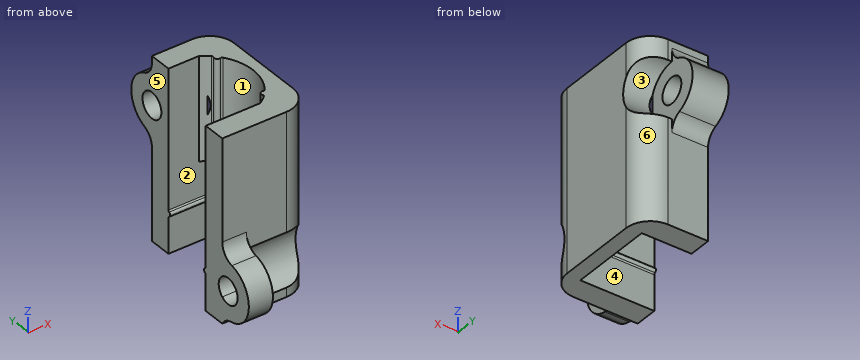
from build123d import *
from build123d.topology import SkipClean

# Parameters (mm, degrees)
SKETCH_1_W          = 8
SKETCH_1_H          = 20
EXTRUDE_1_DEPTH     = 16
CUT_EXTRUDE_1_REACH = 28.833
SKETCH_2_W          = 6.8
SKETCH_2_H          = 10.4
EXTRUDE_3_DEPTH     = 10.8
CUT_EXTRUDE_2_REACH = 28.833
SKETCH_4_R          = 1.6
EXTRUDE_5_DEPTH     = 3
EXTRUDE_START       = -4.5
SKETCH_5_R          = 1.6
EXTRUDE_4_DEPTH     = 4.5
EXTRUDE_START_2     = -3
SKETCH_7_R          = 3.5
SKETCH_7_R_2        = 1.6
EXTRUDE_6_DEPTH     = 3
CUT_EXTRUDE_3_REACH = 31.056
SKETCH_8_R          = 3.5
EXTRUDE_7_DEPTH     = 0.5
CUT_EXTRUDE_4_REACH = 31.27
SKETCH_10_R         = 3.5
EXTRUDE_START_3     = 2
EXTRUDE_8_DEPTH     = 2
FILLET_1_R          = 2
FILLET_2_R          = 3
SKETCH_12_W         = 9.7
SKETCH_12_H         = 10.4
EXTRUDE_9_DEPTH     = 0.6
SKETCH_13_R         = 0.4
EXTRUDE_10_DEPTH    = 12.8
FILLET_3_R          = 0.2
EXTRUDE_11_REACH    = 32.356
SKETCH_14_R         = 0.3
SKETCH_15_R         = 0.3
CUT_EXTRUDE_5_DEPTH = 3
FILLET_4_R          = 0.2


with BuildPart() as part:
    # 草图1 → 凸台-拉伸1 (new body)
    with BuildSketch(Plane(origin=(0, 0, 0), x_dir=(1, 0, 0), z_dir=(0, 1, 0))):
        with Locations((4, 10)):
            Rectangle(SKETCH_1_W, SKETCH_1_H)
    extrude(amount=EXTRUDE_1_DEPTH)

    # 草图2 → 切除-拉伸1 (cut, up to next)
    with BuildSketch(Plane.XY, mode=Mode.PRIVATE) as cut_extrude_1_sk1:
        with Locations((3.4, 8)):
            Rectangle(SKETCH_2_W, SKETCH_2_H)
    cut_extrude_1_tool1 = extrude(cut_extrude_1_sk1.sketch, amount=-CUT_EXTRUDE_1_REACH, mode=Mode.PRIVATE) & part.part
    add(cut_extrude_1_tool1.solids().sort_by_distance((3.4, 8, 0))[0], mode=Mode.SUBTRACT)

    # 草图3 → 凸台-拉伸3 (add)
    with BuildSketch(Plane.XY):
        with BuildLine():
            Line((3.789043744, 13.2), (6.8, 13.2))
            Line((6.8, 13.2), (6.8, 2.8))
            Line((6.8, 2.8), (3.789043744, 2.8))
            ThreePointArc((3.789043744, 2.8), (6.7, 8), (3.789043744, 13.2))
        make_face()
    extrude(amount=-EXTRUDE_3_DEPTH)

    # 草图4 → 切除-拉伸2 (cut, up to next)
    with BuildSketch(Plane(origin=(8, 0, 0), x_dir=(0, 0, -1), z_dir=(1, 0, 0)), mode=Mode.PRIVATE) as cut_extrude_2_sk1:
        with Locations((4, 16)):
            Circle(SKETCH_4_R)
    cut_extrude_2_tool1 = extrude(cut_extrude_2_sk1.sketch, amount=-CUT_EXTRUDE_2_REACH, mode=Mode.PRIVATE) & part.part
    # 草图4 → 切除-拉伸2 (cut, up to next)
    with BuildSketch(Plane(origin=(8, 0, 0), x_dir=(0, 0, -1), z_dir=(1, 0, 0)), mode=Mode.PRIVATE) as cut_extrude_2_sk2:
        with Locations((16, -1)):
            Circle(SKETCH_4_R)
    cut_extrude_2_tool2 = extrude(cut_extrude_2_sk2.sketch, amount=-CUT_EXTRUDE_2_REACH, mode=Mode.PRIVATE) & part.part
    add(cut_extrude_2_tool1.solids().sort_by_distance((8, 16, -4))[0], mode=Mode.SUBTRACT)
    add(cut_extrude_2_tool2.solids().sort_by_distance((8, -1, -16))[0], mode=Mode.SUBTRACT)

    # 草图6 → 凸台-拉伸5 (add)
    with BuildSketch(Plane.ZY):
        with BuildLine():
            Line((-20, 0), (-17.2489996, 0))
            ThreePointArc((-17.2489996, 0), (-16, 0.6), (-14.7510004, 0))
            Line((-14.7510004, 0), (0, 0))
            Line((0, 0), (0, 2.8))
            Line((0, 2.8), (-20, 2.8))
            Line((-20, 2.8), (-20, 0))
        make_face()
    extrude(amount=EXTRUDE_5_DEPTH)

    # 草图5 → 凸台-拉伸4 (add)
    with BuildSketch(Plane.ZY.offset(EXTRUDE_START)):
        with BuildLine():
            Line((-6.1, 13.2), (-1.9, 13.2))
            ThreePointArc((-1.9, 13.2), (-4, 19.5), (-6.1, 13.2))
        make_face()
        with Locations(Location((-4, 16, 0), (0, 0, 180))):
            Circle(SKETCH_5_R, mode=Mode.SUBTRACT)
    extrude(amount=EXTRUDE_4_DEPTH)

    # 草图7 → 凸台-拉伸6 (add)
    with BuildSketch(Plane.ZY.offset(3).offset(EXTRUDE_START_2)):
        with Locations((-16, -1)):
            Circle(SKETCH_7_R)
        with Locations(Location((-16, -1, 0), (0, 0, 141.317812547))):
            Circle(SKETCH_7_R_2, mode=Mode.SUBTRACT)
    extrude(amount=EXTRUDE_6_DEPTH)

    # 草图8 → 切除-拉伸3 (cut, up to next)
    with BuildSketch(Plane(origin=(0, 0, 0), x_dir=(0, 0, -1), z_dir=(1, 0, 0)), mode=Mode.PRIVATE) as cut_extrude_3_sk1:
        with Locations((16, -1)):
            Circle(SKETCH_8_R)
    cut_extrude_3_tool1 = extrude(cut_extrude_3_sk1.sketch, amount=CUT_EXTRUDE_3_REACH, mode=Mode.PRIVATE) & part.part
    add(cut_extrude_3_tool1.solids().sort_by_distance((0, -1, -16))[0], mode=Mode.SUBTRACT)

    # 草图9 → 凸台-拉伸7 (add)
    with SkipClean():  # the faces are left unmerged after this step: merging them gives an invalid solid
        with BuildSketch(Plane(origin=(0, 0, -20), x_dir=(-1, 0, 0), z_dir=(0, 0, -1))):
            Polygon((-6.8, 2.8), (-6.8, 13.2), (0, 13.2), (0, 16), (-8, 16), (-8, 0), (3, 0), (3, 2.8), align=None)
        extrude(amount=EXTRUDE_7_DEPTH)

    # 草图10 → 切除-拉伸4 (cut, up to next)
    with BuildSketch(Plane(origin=(4.5, 0, 0), x_dir=(0, 0, -1), z_dir=(1, 0, 0)), mode=Mode.PRIVATE) as cut_extrude_4_sk1:
        with Locations((4, 16)):
            Circle(SKETCH_10_R)
    cut_extrude_4_tool1 = extrude(cut_extrude_4_sk1.sketch, amount=CUT_EXTRUDE_4_REACH, mode=Mode.PRIVATE) & part.part
    add(cut_extrude_4_tool1.solids().sort_by_distance((4.5, 16, -4))[0], mode=Mode.SUBTRACT)

    # 草图11 → 凸台-拉伸8 (add)
    with SkipClean():  # the faces are left unmerged after this step: merging them gives an invalid solid
        with BuildSketch(Plane.XY.offset(EXTRUDE_START_3)):
            with BuildLine():
                Line((0, 13.2), (3.789043744, 13.2))
                ThreePointArc((3.789043744, 13.2), (6.7, 8), (3.789043744, 2.8))
                Line((3.789043744, 2.8), (-3, 2.8))
                Line((-3, 2.8), (-3, 0))
                Line((-3, 0), (8, 0))
                Line((8, 0), (8, 16))
                Line((8, 16), (0, 16))
                Line((0, 16), (0, 13.2))
            make_face()
        extrude(amount=-EXTRUDE_8_DEPTH)

    # 圆角1
    # the kernel refuses this fillet: 2 mm, written as the material it adds along each edge
    with BuildSketch(Plane(origin=(-3, 0, -19.354101966), x_dir=(0, 0, -1), z_dir=(1, 0, 0))) as fillet_1_piece_1:
        with BuildLine():
            CenterArc((2.09291543, -1.761578284), FILLET_1_R, 118.262295856, 53.77845338)
            ThreePointArc((0.112181831, -1.484640726), (0.135948895, -0.736286166), (0, 0))
            Line((0, 0), (1.145898034, 0))
        make_face()
    extrude(amount=3)
    with BuildSketch(Plane(origin=(-3, 0, -12.645898034), x_dir=(0, 0, 1), z_dir=(1, 0, 0))) as fillet_1_piece_2:
        with BuildLine():
            CenterArc((2.054224947, 2), FILLET_1_R, 190.475681696, 79.524318304)
            ThreePointArc((0.087560615, 1.636363636), (0.140898096, 0.812985117), (0, 0))
            Line((0, 0), (2.054224947, 0))
        make_face()
    extrude(amount=3)
    with BuildSketch(Plane(origin=(0, 16, -7.5), x_dir=(0, 0, -1), z_dir=(1, 0, 0))) as fillet_1_piece_3:
        with BuildLine():
            CenterArc((1.623475383, 2), FILLET_1_R, 201.323686263, 68.676313737)
            ThreePointArc((-0.239606574, 1.272727273), (-0.06042321, 0.647542667), (0, 0))
            Line((0, 0), (1.623475383, 0))
        make_face()
    extrude(amount=4.5)
    with BuildSketch(Plane(origin=(0, 16, -0.5), x_dir=(0, 0, 1), z_dir=(1, 0, 0))) as fillet_1_piece_4:
        with BuildLine():
            CenterArc((1.623475383, -2), FILLET_1_R, 90, 68.676313737)
            ThreePointArc((-0.239606574, -1.272727273), (-0.06042321, -0.647542667), (0, 0))
            Line((0, 0), (1.623475383, 0))
        make_face()
    extrude(amount=4.5)

    # 圆角2
    # the kernel refuses this fillet: 3 mm, written as the material it takes off along each edge
    with BuildSketch(Plane(origin=(8, 16, -8), x_dir=(-1, 0, 0), z_dir=(0, 0, 1))) as fillet_2_piece_1:
        with BuildLine():
            CenterArc((FILLET_2_R, FILLET_2_R), FILLET_2_R, 180, 90)
            Line((0, FILLET_2_R), (0, 0))
            Line((0, 0), (FILLET_2_R, 0))
        make_face()
    extrude(amount=17.5, mode=Mode.SUBTRACT)
    with BuildSketch(Plane(origin=(8, 0, -11.854101966), x_dir=(0, 1, 0), z_dir=(0, 0, -1))) as fillet_2_piece_2:
        with BuildLine():
            CenterArc((FILLET_2_R, -FILLET_2_R), FILLET_2_R, 90, 90)
            Line((0, -FILLET_2_R), (0, 0))
            Line((0, 0), (FILLET_2_R, 0))
        make_face()
    extrude(amount=16.145898034, mode=Mode.SUBTRACT)
    with BuildSketch(Plane(origin=(8, 16, -28), x_dir=(0, -1, 0), z_dir=(0, 0, 1))) as fillet_2_piece_3:
        with BuildLine():
            CenterArc((FILLET_2_R, -FILLET_2_R), FILLET_2_R, 90, 90)
            Line((0, -FILLET_2_R), (0, 0))
            Line((0, 0), (FILLET_2_R, 0))
        make_face()
    extrude(amount=28, mode=Mode.SUBTRACT)
    with BuildSketch(Plane(origin=(8, 0, -20.145898034), x_dir=(0, 1, 0), z_dir=(0, 0, 1))) as fillet_2_piece_4:
        with BuildLine():
            CenterArc((FILLET_2_R, FILLET_2_R), FILLET_2_R, 180, 90)
            Line((0, FILLET_2_R), (0, 0))
            Line((0, 0), (FILLET_2_R, 0))
        make_face()
    extrude(amount=29.645898034, mode=Mode.SUBTRACT)

    # 草图12 → 凸台-拉伸9 (add)
    with BuildSketch(Plane.ZY.offset(-6.8)):
        with Locations((-15.65, 8)):
            Rectangle(SKETCH_12_W, SKETCH_12_H)
    extrude(amount=EXTRUDE_9_DEPTH)

    # 草图13 → 凸台-拉伸10 (add)
    with BuildSketch(Plane.XY.offset(2)):
        with Locations((5.205431576, 12)):
            Circle(SKETCH_13_R)
        with Locations((5.205431576, 4)):
            Circle(SKETCH_13_R)
    extrude(amount=-EXTRUDE_10_DEPTH)

    # 圆角3
    fillet_3_edges = [part.edges().sort_by_distance(p)[0] for p in [
        (4.933376021, 12.293233311, -5.4),
        (5.457684147, 11.689567011, -5.4),
        (5.457684147, 4.310432989, -5.4),
        (4.933376021, 3.706766689, -5.4),
    ]]
    fillet(fillet_3_edges, radius=FILLET_3_R)

    # 凸台-拉伸11: up to this face of the body (flat: up to its plane)
    extrude_11_end = Plane(part.part.faces().sort_by_distance((6.2, 8, -15.65))[0])
    # 草图14 → 凸台-拉伸11 (add, up to the picked face)
    with BuildSketch(Plane.ZY.offset(3), mode=Mode.PRIVATE) as extrude_11_sk1:
        with Locations((-15.65, 13.2)):
            Circle(SKETCH_14_R)
    extrude_11_tool1 = split(extrude(extrude_11_sk1.sketch, amount=-EXTRUDE_11_REACH, mode=Mode.PRIVATE), bisect_by=extrude_11_end, keep=Keep.BOTH, mode=Mode.PRIVATE)
    # 草图14 → 凸台-拉伸11 (add, up to the picked face)
    with BuildSketch(Plane.ZY.offset(3), mode=Mode.PRIVATE) as extrude_11_sk2:
        with Locations((-15.65, 2.8)):
            Circle(SKETCH_14_R)
    extrude_11_tool2 = split(extrude(extrude_11_sk2.sketch, amount=-EXTRUDE_11_REACH, mode=Mode.PRIVATE), bisect_by=extrude_11_end, keep=Keep.BOTH, mode=Mode.PRIVATE)
    add(extrude_11_tool1.solids().sort_by(Axis((-3, 13.2, -15.65), (1, 0, 0)))[0])
    add(extrude_11_tool2.solids().sort_by(Axis((-3, 2.8, -15.65), (1, 0, 0)))[0])

    # 草图15 → 切除-拉伸5 (cut)
    with BuildSketch(Plane.ZY.offset(3)):
        with Locations((-15.65, 13.2)):
            Circle(SKETCH_15_R)
    extrude(amount=-CUT_EXTRUDE_5_DEPTH, mode=Mode.SUBTRACT)

    # 圆角4
    # the kernel refuses this fillet: 0.2 mm, written as the material it adds along each edge
    with BuildSketch(Plane(origin=(6.595643924, 13.2, -15.95), x_dir=(0, -0.978906312930706, 0.20430964368920726), z_dir=(-1, 0, 0))) as fillet_4_piece_1:
        with BuildLine():
            CenterArc((0.163447715, -0.195781263), FILLET_4_R, 101.789089239, 66.421821522)
            Line((-0.032333548, -0.154919334), (0, 0))
            ThreePointArc((0, 0), (0.061292893, -0.006328106), (0.122585786, 0))
        make_face()
    extrude(amount=6.595643924)
    with BuildSketch(Plane(origin=(0, 13.2, -15.35), x_dir=(0, 0, 1), z_dir=(1, 0, 0))) as fillet_4_piece_2:
        with BuildLine():
            CenterArc((0.158257569, 0.2), FILLET_4_R, 203.578178478, 66.421821522)
            ThreePointArc((-0.025045458, 0.12), (-0.006328106, 0.061292893), (0, 0))
            Line((0, 0), (0.158257569, 0))
        make_face()
    extrude(amount=6.595643924)
    with BuildSketch(Plane(origin=(-3, 2.8, -15.35), x_dir=(0, 0, 1), z_dir=(1, 0, 0))) as fillet_4_piece_3:
        with BuildLine():
            CenterArc((0.158257569, -0.2), FILLET_4_R, 90, 66.421821522)
            ThreePointArc((-0.025045458, -0.12), (-0.006328106, -0.061292893), (0, 0))
            Line((0, 0), (0.158257569, 0))
        make_face()
    extrude(amount=9.595643924)
    with BuildSketch(Plane(origin=(6.595643924, 2.8, -15.95), x_dir=(0, 0.9789063129307064, 0.20430964368920507), z_dir=(-1, 0, 0))) as fillet_4_piece_4:
        with BuildLine():
            CenterArc((0.163447715, 0.195781263), FILLET_4_R, 191.789089239, 66.421821522)
            Line((-0.032333548, 0.154919334), (0, 0))
            ThreePointArc((0, 0), (0.061292893, 0.006328106), (0.122585786, 0))
        make_face()
    extrude(amount=9.595643924)


solid = part.part
The model under review builds one solid part; all positions refer to its coordinate system, in mm. Face numbers are marked on the shaded views. A direction names the side the tool comes from. Coordinates: 2 decimals unless noted, no trailing zeros. Write each loop counter-clockwise with the first axis right and the second up, starting at its lowest first coordinate (ties: lowest second). Pieces come first, ordered by that corner, then holes. Notation, with made-up numbers: (-38, 68) -> (15, 68) arc R28 ccw to (15, 90) -> close; hole circle Ø2 at (17.5, 34). An arc over 180 degrees is marked (long way). Answer in a Markdown table with one row per item.
1. Clearance check with flat-ended pins moving along their axes: pin 1 Ø1.9 at (x, y) = (5, 11.5) entering from -Z; pin 2 Ø6 at (x, z) = (3, -9.5) entering from +Y; pin 3 Ø5 at (y, z) = (-1, -16) entering from +X; pin 4 Ø0.6 at (x, y) = (6.5, 9) entering from +Z. State where each tip first meets the part, or that it passes through.
Answers below:
| item | result |
|---|---|
| pin 1 | stops at z = -10.8 |
| pin 2 | stops at y = 18.45 |
| pin 3 | stops at x = 0 |
| pin 4 | stops at z = 2 |
2. Draft analysis for pull direction Y (two halves, no side actions). For the marked faces 4, 5 and 6, state which applies: +Y half, -Y half, draft (parallel to the pull), parting line (faces both ways), or undercut.
Answers below:
| item | result |
|---|---|
| face 4 | undercut |
| face 5 | draft |
| face 6 | +Y half |
3. We need section D-D, the plane y = 13.5. State the section outline as (x, z) points.
Answers below:
| item | result |
|---|---|
| outline | (0, -20.5) -> (7.96, -20.5) -> (7.96, -6.45) -> (4.5, -6.45) -> (4.5, -1.55) -> (7.96, -1.55) -> (7.96, 2) -> (0, 2) -> close |
4. We need section B-B, the plane x = -2. State the section outline as (y, z) points.
Answers below:
| item | result |
|---|---|
| outline | (-1.64, -12.56) arc R3.5 ccw to (-1.48, -19.47) arc R2 cw to (0, -20.5) -> (2.8, -20.5) -> (2.8, -16.11) arc R0.2 cw to (2.92, -15.92) arc R0.3 ccw to (2.92, -15.38) arc R0.2 cw to (2.8, -15.19) -> (2.8, 2) -> (0, 2) -> (0, -10.59) arc R2 cw to start; hole circle Ø3.2 at (-1, -16) |
5. We need section A-A, the plane x = 2.5. State the section outline as (y, z) points, and give its area (3 significant figures).
Answers below:
| item | result |
|---|---|
| outline | (0, -20.5) -> (2.8, -20.5) -> (2.8, -16.11) arc R0.2 cw to (2.92, -15.92) arc R0.3 ccw to (2.92, -15.38) arc R0.2 cw to (2.8, -15.19) -> (2.8, 2) -> (0, 2) -> (0, -12.65) arc R3.5 cw to (0, -19.35) -> close; (13.08, -15.92) arc R0.2 cw to (13.2, -16.11) -> (13.2, -20.5) -> (16, -20.5) -> (16, -9.12) arc R2 cw to (17.27, -7.26) arc R3.5 ccw to (17.27, -0.74) arc R2 cw to (16, 1.12) -> (16, 2) -> (13.2, 2) -> (13.2, -15.19) arc R0.2 cw to (13.08, -15.38) arc R0.3 ccw to start; hole circle Ø3.2 at (16, -4) |
| area | 126 mm^2 |
6. We need section C-C, the plane y = -1. State the section outline as (x, z) points, and give its area (3 significant figures).
Answers below:
| item | result |
|---|---|
| outline | (-3, -19.6) -> (0, -19.6) -> (0, -17.6) -> (-3, -17.6) -> close; (-3, -14.4) -> (0, -14.4) -> (0, -12.32) -> (-3, -12.32) -> close |
| area | 12.2 mm^2 |
7. Wall thickness on probe 1 along Y at (x, z) = (2.5, -12.5); probe 2 along X at (y, z) = (16, -7); probe 3 along Y at (x, z) = (-1.5, 1): over which ranges is each line inside the solid? List them lowest first. Write a range as [from, to].
Answers below:
| item | result |
|---|---|
| probe 1 | y = [0, 2.8], [13.2, 16] |
| probe 2 | x = [0, 4.5] |
| probe 3 | y = [0, 2.8] |
8. For the marked faces 1, 2 and 3, list the 3-axis set-ups (+Z, -Z, +X, -X, +Y, -Y) from which the entire face can be reached by the end or side of a thin tool; tool diameter is ignored.
Answers below:
| item | result |
|---|---|
| face 1 | +Z, -X |
| face 2 | -X |
| face 3 | +X, +Y |
